from build123d import *

# Parameters (mm, degrees)
SKETCH_1_W          = 133
SKETCH_1_H          = 50
EXTRUDE_1_DEPTH     = 2
FILLET_1_R          = 3
SKETCH_2_R          = 1.6
CUT_EXTRUDE_1_DEPTH = 3
SKETCH_3_W          = 43.714876359
SKETCH_3_H          = 21.542228592
CUT_EXTRUDE_2_DEPTH = 10
SKETCH_4_W          = 83
SKETCH_4_H          = 15
CUT_EXTRUDE_3_DEPTH = 10
FILLET_3_R          = 3
FILLET_4_R          = 3


with BuildPart() as part:
    # 草图1 → 凸台-拉伸1 (new body)
    with BuildSketch(Plane.XY):
        Rectangle(SKETCH_1_W, SKETCH_1_H)
    extrude(amount=EXTRUDE_1_DEPTH)

    # 圆角1
    fillet_1_edges = [part.edges().sort_by_distance(p)[0] for p in [
        (-66.5, 25, 1),
        (66.5, 25, 1),
        (66.5, -25, 1),
        (-66.5, -25, 1),
    ]]
    fillet(fillet_1_edges, radius=FILLET_1_R)

    # 草图2 → 切除-拉伸1 (cut)
    with BuildSketch(Plane.XY.offset(2)):
        with Locations((-60.5, 10)):
            Circle(SKETCH_2_R)
        with Locations((-60.5, -10)):
            Circle(SKETCH_2_R)
        with Locations((60.5, -10)):
            Circle(SKETCH_2_R)
        with Locations((60.5, 10)):
            Circle(SKETCH_2_R)
    extrude(amount=-CUT_EXTRUDE_1_DEPTH, mode=Mode.SUBTRACT)

    # 草图3 → 切除-拉伸2 (cut)
    with BuildSketch(Plane.XY.offset(2)):
        with BuildLine():
            Line((-50.5, 20), (-50.5, 0))
            ThreePointArc((-50.5, 0), (-52.5, -2), (-54.5, 0))
            Line((-54.5, 0), (-54.5, 20))
            ThreePointArc((-54.5, 20), (-52.5, 22), (-50.5, 20))
        make_face()
        with BuildLine():
            Line((-46.5, 20), (-46.5, 0))
            ThreePointArc((-46.5, 0), (-44.5, -2), (-42.5, 0))
            Line((-42.5, 0), (-42.5, 20))
            ThreePointArc((-42.5, 20), (-44.5, 22), (-46.5, 20))
        make_face()
        with BuildLine():
            Line((-38.5, 20), (-38.5, 0))
            ThreePointArc((-38.5, 0), (-36.5, -2), (-34.5, 0))
            Line((-34.5, 0), (-34.5, 20))
            ThreePointArc((-34.5, 20), (-36.5, 22), (-38.5, 20))
        make_face()
        with BuildLine():
            Line((-30.5, 20), (-30.5, 0))
            ThreePointArc((-30.5, 0), (-28.5, -2), (-26.5, 0))
            Line((-26.5, 0), (-26.5, 20))
            ThreePointArc((-26.5, 20), (-28.5, 22), (-30.5, 20))
        make_face()
        with Locations((-0.774062545, 10.771114296)):
            Rectangle(SKETCH_3_W, SKETCH_3_H)
        with BuildLine():
            Line((25.5, 20), (25.5, 0))
            ThreePointArc((25.5, 0), (27.5, -2), (29.5, 0))
            Line((29.5, 0), (29.5, 20))
            ThreePointArc((29.5, 20), (27.5, 22), (25.5, 20))
        make_face()
        with BuildLine():
            Line((33.5, 20), (33.5, 0))
            ThreePointArc((33.5, 0), (35.5, -2), (37.5, 0))
            Line((37.5, 0), (37.5, 20))
            ThreePointArc((37.5, 20), (35.5, 22), (33.5, 20))
        make_face()
        with BuildLine():
            Line((41.5, 20), (41.5, 0))
            ThreePointArc((41.5, 0), (43.5, -2), (45.5, 0))
            Line((45.5, 0), (45.5, 20))
            ThreePointArc((45.5, 20), (43.5, 22), (41.5, 20))
        make_face()
        with BuildLine():
            Line((49.5, 20), (49.5, 0))
            ThreePointArc((49.5, 0), (51.5, -2), (53.5, 0))
            Line((53.5, 0), (53.5, 20))
            ThreePointArc((53.5, 20), (51.5, 22), (49.5, 20))
        make_face()
    extrude(amount=-CUT_EXTRUDE_2_DEPTH, mode=Mode.SUBTRACT)

    # 草图4 → 切除-拉伸3 (cut)
    with BuildSketch(Plane.XY.offset(2)):
        with Locations((0, -17.5)):
            Rectangle(SKETCH_4_W, SKETCH_4_H)
    extrude(amount=-CUT_EXTRUDE_3_DEPTH, mode=Mode.SUBTRACT)

    # 圆角3
    fillet_3_edges = [part.edges().sort_by_distance(p)[0] for p in [
        (-41.5, -25, 1),
        (-41.5, -10, 1),
        (41.5, -10, 1),
        (41.5, -25, 1),
    ]]
    fillet(fillet_3_edges, radius=FILLET_3_R)

    # 圆角4
    fillet_4_edges = [part.edges().sort_by_distance(p)[0] for p in [
        (-22.631500725, 0, 1),
        (-22.631500725, 21.542228592, 1),
        (21.083375634, 21.542228592, 1),
        (21.083375634, 0, 1),
    ]]
    fillet(fillet_4_edges, radius=FILLET_4_R)


solid = part.part
CAD build for the part. Positions are in the model's coordinates, mm. A direction names the side the tool comes from. Give positions to 0.01 mm unless a question says otherwise; leave off trailing zeros. Loops run counter-clockwise (first coordinate to the right, second up) from the corner with the lowest first, then second, coordinate; pieces in that order, holes last. Notation, with made-up numbers: M -38,33 L -23,33 A25 ccw -23,45 Z; hole C -28,78 d5. An arc over 180 degrees is marked long. Answer in a Markdown table with one row per item. Add a question column.
Item 1: Band-saw the part on D-D on y = 10. Give the number of separate pieces and of enclosed holes in the cut face, then the cut area to 3 significant figures.
Item 2: Band-saw the part on B-B on x = -7. Give the cut face in (y, z), then the cut area to 3 significant figures.
Item 3: Mould opens along X. For faces 1 (the face through (20.23, 20.64, 0.99)), 2 (the face through (65.64, 24.1, 1.01)), 3 (the face through (-59.02, 9.39, 1.01)), 4 (the face through (-65.64, -24.1, 1.01)) say: +X half, -X half, draft (parallel to the pull), parting line (faces both ways), or undercut.
Item 4: Band-saw the part on C-C on y = -20.5. Give the cut face in (x, z).
Item 5: Tool access for faces 5 (the face through (42.4, -24.14, 0.99)), 6 (the face through (-1, -5, 0)), 7 (the face through (-21.776, 20.64, 0.986)): list every direction of +Z, -Z, +X, -X, +Y, -Y with a clear straight run to the whole face (end or side of a thin tool).
Item 6: Probe probe 1 along Y at (x, z) = (-60.5, 1); probe 2 along Y at (x, z) = (-17, 0.5); probe 3 along X at (y, z) = (-19.5, 1.4). List the from-to ranges inside material, lowest first.
Item 7: Drop flat-ended pins along their axis: P1, Ø1.9, axis at x = -60.5, y = -10, coming from the +Z side; P2, Ø0.6, axis at x = 2, z = 1.5, coming from the -Y side. Give the stop position or say it passes through.
Item 8: Band-saw the part on A-A on x = 60.5. Give the cut face in (y, z), then the cut area to 3 significant figures.
Reply:
| question | item | result |
|---|---|---|
| 1 | separate pieces | 12 |
| 1 | enclosed holes | 0 |
| 1 | area | 102 mm^2 |
| 2 | outline | M -10,0 L 0,0 L 0,2 L -10,2 Z; M 21.54,0 L 25,0 L 25,2 L 21.54,2 Z |
| 2 | area | 26.9 mm^2 |
| 3 | face 1 | undercut |
| 3 | face 2 | +X half |
| 3 | face 3 | undercut |
| 3 | face 4 | -X half |
| 4 | outline | M -66.5,0 L -41.5,0 L -41.5,2 L -66.5,2 Z; M 41.5,0 L 66.5,0 L 66.5,2 L 41.5,2 Z |
| 5 | face 5 | +Z, -Z, -Y |
| 5 | face 6 | -Z, +X, -X, +Y, -Y |
| 5 | face 7 | +Z, -Z |
| 6 | probe 1 | y = -25 to -11.6, -8.4 to 8.4, 11.6 to 25 |
| 6 | probe 2 | y = -10 to 0, 21.54 to 25 |
| 6 | probe 3 | x = -66.5 to -41.5, 41.5 to 66.5 |
| 7 | P1 | passes through |
| 7 | P2 | stops at y = -10 |
| 8 | outline | M -25,0 L -11.6,0 L -11.6,2 L -25,2 Z; M -8.4,0 L 8.4,0 L 8.4,2 L -8.4,2 Z; M 11.6,0 L 25,0 L 25,2 L 11.6,2 Z |
| 8 | area | 87.2 mm^2 |
